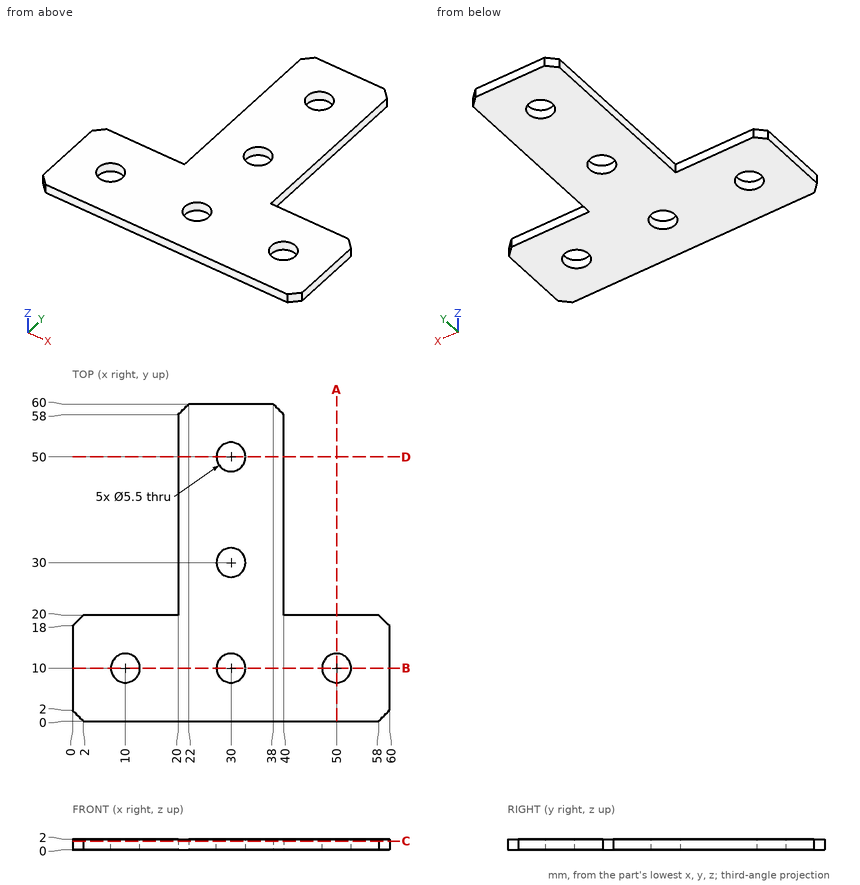
For this review, use the dimensioned drawing (mm, ordinates from the lowest corner) and the shaded views. Coordinates: 2 decimals unless noted, no trailing zeros. Loops run counter-clockwise (first coordinate to the right, second up) from the corner with the lowest first, then second, coordinate; pieces in that order, holes last. Notation, with made-up numbers: (37.25, 0.5) -> (59.25, 0.5) arc R27 cw to (59.25, 16.5) -> close; hole circle Ø2 at (19, 23). An arc over 180 degrees is marked (long way). Use a Markdown table: item, result. Add a question column.
Item 1: We need section C-C, the plane z = 1.6. Write out the cut boundary in (x, y).
Item 2: We need section B-B, the plane y = 10. Write out the cut boundary in (x, z).
Item 3: We need section D-D, the plane y = 50. Write out the cut boundary in (x, z).
Item 4: We need section A-A, the plane x = 50. Write out the cut boundary in (y, z).
Item 5: Clearance check with flat-ended pins moving along their axes: P1, Ø6.5, axis at x = 50, y = 10, coming from the -Z side; P2, Ø0.6, axis at y = 32.5, z = 1, coming from the -X side; P3, Ø0.6, axis at x = 46, z = 1, coming from the +Y side. State where each tip first meets the part, or that it passes through.
Item 6: Wall thickness on L1, parallel to Y at x = 30, z = 1.5; L2, parallel to X at y = 50, z = 0.75: over which ranges is each line inside the solid? List them lowest first. Write a range as from..to.
Numbers:
| question | item | result |
|---|---|---|
| 1 | outline | (0, 2) -> (2, 0) -> (58, 0) -> (60, 2) -> (60, 18) -> (58, 20) -> (40, 20) -> (40, 58) -> (38, 60) -> (22, 60) -> (20, 58) -> (20, 20) -> (2, 20) -> (0, 18) -> close; hole circle Ø5.5 at (10, 10); hole circle Ø5.5 at (30, 10); hole circle Ø5.5 at (30, 30); hole circle Ø5.5 at (30, 50); hole circle Ø5.5 at (50, 10) |
| 2 | outline | (0, 0) -> (7.25, 0) -> (7.25, 2) -> (0, 2) -> close; (12.75, 0) -> (27.25, 0) -> (27.25, 2) -> (12.75, 2) -> close; (32.75, 0) -> (47.25, 0) -> (47.25, 2) -> (32.75, 2) -> close; (52.75, 0) -> (60, 0) -> (60, 2) -> (52.75, 2) -> close |
| 3 | outline | (20, 0) -> (27.25, 0) -> (27.25, 2) -> (20, 2) -> close; (32.75, 0) -> (40, 0) -> (40, 2) -> (32.75, 2) -> close |
| 4 | outline | (0, 0) -> (7.25, 0) -> (7.25, 2) -> (0, 2) -> close; (12.75, 0) -> (20, 0) -> (20, 2) -> (12.75, 2) -> close |
| 5 | P1 | stops at z = 0 |
| 5 | P2 | stops at x = 20 |
| 5 | P3 | stops at y = 20 |
| 6 | L1 | y = 0..7.25, 12.75..27.25, 32.75..47.25, 52.75..60 |
| 6 | L2 | x = 20..27.25, 32.75..40 |
